Can you work these out from the model? Positions are in its coordinate system, mm. Face numbers are marked on the shaded views. Round coordinates to 2 decimals unless told otherwise and drop trailing zeros. Loops run counter-clockwise (first coordinate to the right, second up) from the corner with the lowest first, then second, coordinate; pieces in that order, holes last. Notation, with made-up numbers: (66, -39.75) - (82, -39.75) arc R17 ccw to (82, -32.75) - close; hole circle Ø4 at (-13.75, -27.5). An arc over 180 degrees is marked (long way). Answer as CSV lines item,"result".
```python
from build123d import *

# Parameters (mm, degrees)
F1_DEPTH = 10
F3_D     = 9
F4_R     = 19.1
F5_DEPTH = 10


with BuildPart() as f1:
    # F0 (on Top) → F1 (new body)
    with BuildSketch(Plane.XY):
        with BuildLine():
            Line((-15.5344827586, 21.4692767792), (-34.5689655172, 7.696533185))
            ThreePointArc((-34.5689655172, 7.696533185), (-38.5, 0), (-34.5689655172, -7.696533185))
            Line((-34.5689655172, -7.696533185), (-15.5344827586, -21.4692767792))
            ThreePointArc((-15.5344827586, -21.4692767792), (0, -26.5), (15.5344827586, -21.4692767792))
            Line((15.5344827586, -21.4692767792), (34.5689655172, -7.696533185))
            ThreePointArc((34.5689655172, -7.696533185), (38.5, 0), (34.5689655172, 7.696533185))
            Line((34.5689655172, 7.696533185), (15.5344827586, 21.4692767792))
            ThreePointArc((15.5344827586, 21.4692767792), (0, 26.5), (-15.5344827586, 21.4692767792))
        make_face()
    extrude(amount=F1_DEPTH)

    # F3 (through all)
    with Locations(Plane.XY.offset(10)):
        with Locations((-29, 0), (29, 0)):
            Hole(F3_D / 2)

    # F4 (on face) → F5 (cut, through all)
    with BuildSketch(Plane.XY.offset(10)):
        Circle(F4_R)
    extrude(amount=-F5_DEPTH, mode=Mode.SUBTRACT)


solid = f1.part
```
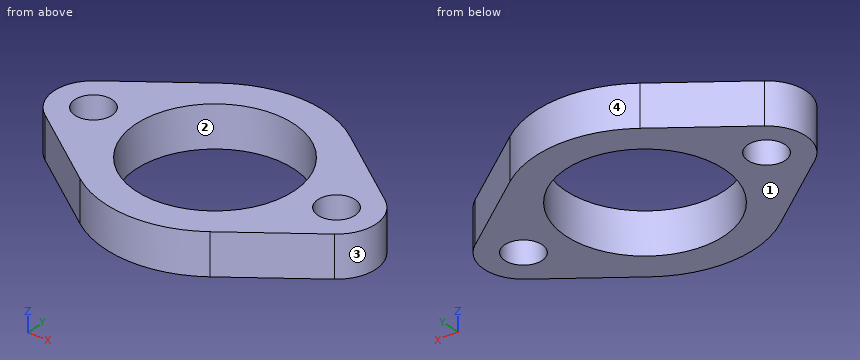
Q1. I'm going to push flat-ended pins straight in: pin 1 Ø5 at (x, y) = (-26, 10.5) entering from -Z; pin 2 Ø2 at (y, z) = (16.5, 7.5) entering from -X; pin 3 Ø4 at (x, z) = (-25.5, 1) entering from +Y; pin 4 Ø4 at (y, z) = (-10.5, 2) entering from -X. Where does each tip first touch, or does it pass through?
Checks:
pin 1,"z = 0"
pin 2,"x = -23.78"
pin 3,"y = 15.71"
pin 4,"x = -33.46"
Q2. Imagine slicing it at B-B (z = 8.5). Write out the boundary of the cut face in (x, y), then the cut area to 3 significant figures.
Checks:
outline,"(-34.57, -7.7) - (-15.53, -21.47) arc R26.5 ccw to (15.53, -21.47) - (34.57, -7.7) arc R9.5 ccw to (34.57, 7.7) - (15.53, 21.47) arc R26.5 ccw to (-15.53, 21.47) - (-34.57, 7.7) arc R9.5 ccw to start; hole circle Ø9 at (-29, 0); hole circle Ø38.2 at (0, 0); hole circle Ø9 at (29, 0)"
area,"1,470 mm²"
Q3. We'd pull the mould along X, two halves only. Please class the marked faces 1, 2, 3 and 4: pulls with the +X half, pulls with the -X half, needs draft (parallel to the pull), parting line crosses it, or undercut.
Checks:
face 1,"needs draft"
face 2,"undercut"
face 3,"pulls with the +X half"
face 4,"parting line crosses it"
Q4. Imagine slicing it at D-D (y = -16.5). Write out the boundary of the cut face in (x, z), then the cut area to 3 significant figures.
Checks:
outline,"(-22.4, 0) - (-9.62, 0) - (-9.62, 10) - (-22.4, 10) - close; (9.62, 0) - (22.4, 0) - (22.4, 10) - (9.62, 10) - close"
area,"256 mm²"
Q5. If I drill on line 1 along X through (y, z) = (-4, 3.75); line 2 along X through (y, z) = (-3, 2); line 3 along Y through (x, z) = (-3.5, 5.5), over which ranges is the centre line in solid material (lowest first)? Write a range as [from, to].
Checks:
line 1,"[-37.62, -31.06], [-26.94, -18.68], [18.68, 26.94], [31.06, 37.62]"
line 2,"[-38.01, -32.35], [-25.65, -18.86], [18.86, 25.65], [32.35, 38.01]"
line 3,"[-26.27, -18.78], [18.78, 26.27]"
Q6. Imagine slicing it at C-C (y = 0). Write out the boundary of the cut face in (x, z), then the cut area to 3 significant figures.
Checks:
outline,"(-38.5, 0) - (-33.5, 0) - (-33.5, 10) - (-38.5, 10) - close; (-24.5, 0) - (-19.1, 0) - (-19.1, 10) - (-24.5, 10) - close; (19.1, 0) - (24.5, 0) - (24.5, 10) - (19.1, 10) - close; (33.5, 0) - (38.5, 0) - (38.5, 10) - (33.5, 10) - close"
area,"208 mm²"
Q7. Imagine slicing it at A-A (x = 0). Write out the boundary of the cut face in (y, z).
Checks:
outline,"(-26.5, 0) - (-19.1, 0) - (-19.1, 10) - (-26.5, 10) - close; (19.1, 0) - (26.5, 0) - (26.5, 10) - (19.1, 10) - close"
